```python
from build123d import *

# Parameters (mm, degrees)
SKETCH1_W           = 125
SKETCH1_H           = 80
BOSS_EXTRUDE1_DEPTH = 2
SKETCH3_W           = 120
SKETCH3_H           = 75
BOSS_EXTRUDE2_DEPTH = 3
SKETCH4_W           = 104.904455421
SKETCH4_H           = 41
CUT_EXTRUDE1_DEPTH  = 3


with BuildPart() as part:
    # Sketch1 → Boss-Extrude1 (new body)
    with BuildSketch(Plane(origin=(0, 0, 0), x_dir=(1, 0, 0), z_dir=(0, 1, 0))):
        with Locations((62.5, 40)):
            Rectangle(SKETCH1_W, SKETCH1_H)
    extrude(amount=BOSS_EXTRUDE1_DEPTH)

    # Sketch3 → Boss-Extrude2 (add)
    with BuildSketch(Plane(origin=(0, 2, 0), x_dir=(1, 0, 0), z_dir=(0, 1, 0))):
        with Locations((62.403820475, 39.836034952)):
            Rectangle(SKETCH3_W, SKETCH3_H)
    extrude(amount=BOSS_EXTRUDE2_DEPTH)

    # Sketch4 → Cut-Extrude1 (cut)
    with BuildSketch(Plane(origin=(0, 5, 0), x_dir=(1, 0, 0), z_dir=(0, 1, 0))):
        with Locations((54.856048186, 39.836034952)):
            Rectangle(SKETCH4_W, SKETCH4_H)
    extrude(amount=-CUT_EXTRUDE1_DEPTH, mode=Mode.SUBTRACT)


solid = part.part
```
Work out the finished part from the listing and answer in its coordinate system (mm). A direction names the side the tool comes from. Give positions to 0.01 mm unless a question says otherwise; leave off trailing zeros. Loops run counter-clockwise (first coordinate to the right, second up) from the corner with the lowest first, then second, coordinate; pieces in that order, holes last. Notation, with made-up numbers: (39, 18) - (72, 18) arc R14 cw to (72, 28) - close; hole circle Ø2 at (14, 49). An arc over 180 degrees is marked (long way). One line per question, with ' | ' between items.
(1) Each of these flat-tipped pins is pushed along its axis until it touches: pin 1 Ø1.5 at (x, y) = (31, 3) entering from +Z; pin 2 Ø8 at (x, z) = (14.5, -45) entering from +Y; pin 3 Ø0.9 at (y, z) = (3, -68) entering from -X. Where does it stop, or does it pass through?
Recorded:
pin 1: stops at z = -2.34 | pin 2: stops at y = 2 | pin 3: stops at x = 2.4
(2) The mould has two halves that part along Z. Classify faces 5 (the face through (122.404, 3, -39)), 6 (the face through (62, 3, -77.336)), 7 (the face through (107.308, 4, -40)), 8 (the face through (62, 2, -41)): +Z half, -Z half, draft (parallel to the pull), parting line (faces both ways), or undercut.
Recorded:
face 5: draft | face 6: -Z half | face 7: undercut | face 8: undercut
(3) The part is cut by section C-C (z = -23). Write down the section's boundary in (x, y).
Recorded:
outline: (0, 0) - (125, 0) - (125, 2) - (122.4, 2) - (122.4, 5) - (107.31, 5) - (107.31, 2) - (0, 2) - close
(4) The part is cut by section A-A (z = -67.5). Write down the section's boundary in (x, y), then the cut area to 3 significant figures.
Recorded:
outline: (0, 0) - (125, 0) - (125, 2) - (122.4, 2) - (122.4, 5) - (2.4, 5) - (2.4, 2) - (0, 2) - close | area: 610 mm²
(5) Straight lines are drawn through the part: probe 1 along Z at (x, y) = (23, 3.5); probe 2 along Y at (x, z) = (85, -42.5); probe 3 along X at (y, z) = (4.1, -74). For each, find the intervals that lie inside material, in ascending order.
Recorded:
probe 1: z = -77.34 to -60.34, -19.34 to -2.34 | probe 2: y = 0 to 2 | probe 3: x = 2.4 to 122.4
(6) A tool of negligible diameter and unlimited length cuts with its end or side. For faces 1 (the face through (62, 0, -41)), 2 (the face through (62, 3, -2.336)), 3 (the face through (54, 4, -19.336)), 4 (the face through (2.404, 3, -11)), from which of +Z, -Z, +X, -X, +Y, -Y can it reach the whole face along a straight path? Write none if from no direction.
Recorded:
face 1: +Z, -Z, +X, -X, -Y | face 2: +Z, +X, -X, +Y | face 3: -X, +Y | face 4: +Z, -Z, -X, +Y
(7) The part is cut by section B-B (x = 66). Write down the section's boundary in (y, z), then the cut area to 3 significant figures.
Recorded:
outline: (0, -80) - (2, -80) - (2, -77.34) - (5, -77.34) - (5, -60.34) - (2, -60.34) - (2, -19.34) - (5, -19.34) - (5, -2.34) - (2, -2.34) - (2, 0) - (0, 0) - close | area: 262 mm²
